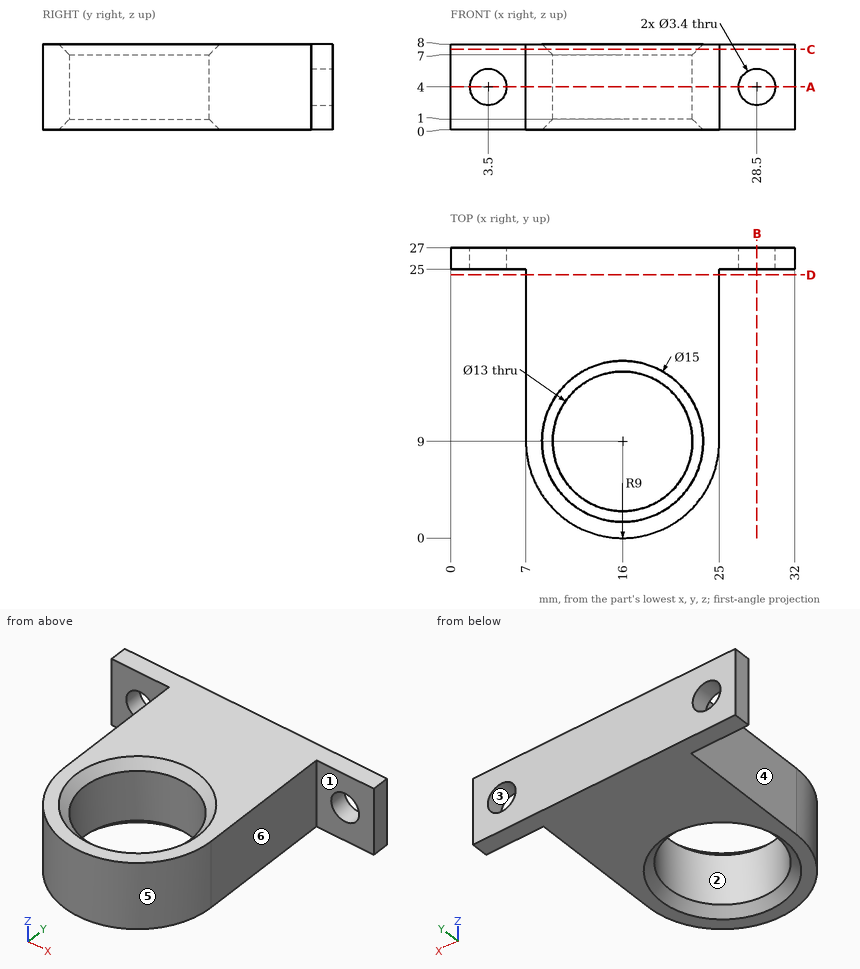
Geometry: see drawing. Coordinates: mm, zero at the bounding-box minimum. A direction names the side the tool comes from. Give positions to 0.01 mm unless a question says otherwise; leave off trailing zeros. Loops run counter-clockwise (first coordinate to the right, second up) from the corner with the lowest first, then second, coordinate; pieces in that order, holes last. Notation, with made-up numbers: (-27.75, 65) - (16.25, 65) arc R22 ccw to (16.25, 71) - close; hole circle Ø7 at (-22.75, 75.5). An arc over 180 degrees is marked (long way). Use CSV: the item, a comma, the result in double quotes.
1) Cut plane C-C (z = 7.5). Output: boundary loops of the cut face in (x, y), and give its area (3 significant figures).
Worked out:
outline,"(0, 25) - (7, 25) - (7, 9) arc R9 ccw to (25, 9) - (25, 25) - (32, 25) - (32, 27) - (0, 27) - close; hole circle Ø14 at (16, 9)"
area,"325 mm^2"
2) Line query: line 1 (X direction, y = 26.3, z = 4); line 2 (Z direction, x = 3.5, y = 25.55); line 3 (Y direction, x = 16, z = 2.85). Output: solid intervals per line, ascending.
Worked out:
line 1,"x = 0 to 1.8, 5.2 to 26.8, 30.2 to 32"
line 2,"z = 0 to 2.3, 5.7 to 8"
line 3,"y = 0 to 2.5, 15.5 to 27"
3) Set-up query: the marked faces 4, 5 and 6. Return all of +Z, -Z, +X, -X, +Y, -Y with unobstructed straight access to the full face (end or side cutting, diameter ignored); none if empty.
Worked out:
face 4,"+Z, -Z, -X, -Y"
face 5,"+Z, -Z, -Y"
face 6,"+Z, -Z, +X, -Y"
4) Cut plane A-A (z = 4). Output: boundary loops of the cut face in (x, y), and give its area (3 significant figures).
Worked out:
outline,"(0, 25) - (1.8, 25) - (1.8, 27) - (0, 27) - close; (5.2, 25) - (7, 25) - (7, 9) arc R9 ccw to (25, 9) - (25, 25) - (26.8, 25) - (26.8, 27) - (5.2, 27) - close; (30.2, 25) - (32, 25) - (32, 27) - (30.2, 27) - close; hole circle Ø13 at (16, 9)"
area,"333 mm^2"
5) Cut plane B-B (x = 28.5). Output: boundary loops of the cut face in (y, z), and give its area (3 significant figures).
Worked out:
outline,"(25, 0) - (27, 0) - (27, 2.3) - (25, 2.3) - close; (25, 5.7) - (27, 5.7) - (27, 8) - (25, 8) - close"
area,"9.20 mm^2"
6) Pin query (flat end, axial travel): P1, Ø2, axis at x = 27.5, z = 4.5, coming from the -Y side; P2, Ø4, axis at y = 13, z = 2.5, coming from the +X side. Return the tip coordinate at first contact, or that it passes through.
Worked out:
P1,"stops at y = 25"
P2,"stops at x = 25"
7) Cut plane D-D (y = 24.5). Output: boundary loops of the cut face in (x, z).
Worked out:
outline,"(7, 0) - (25, 0) - (25, 8) - (7, 8) - close"
8) Mould query, pull axis Y, two halves, no side actions, for the marked faces 1, 2 and 3. Classes: +Y half, -Y half, draft (parallel to the pull), parting line (faces both ways), or undercut.
Worked out:
face 1,"-Y half"
face 2,"undercut"
face 3,"draft"
